CAD build for the part. Positions are in the model's coordinates, mm. A direction names the side the tool comes from. Give positions to 0.01 mm unless a question says otherwise; leave off trailing zeros. Write each loop counter-clockwise with the first axis right and the second up, starting at its lowest first coordinate (ties: lowest second). Pieces come first, ordered by that corner, then holes. Notation, with made-up numbers: (25, -16.75) -> (31, -16.75) arc R21 cw to (31, 13.25) -> close; hole circle Ø4 at (15, 21.5). An arc over 180 degrees is marked (long way). Answer as a JSON object with one key per item and string values.
Autodesk Inventor part; units mm, degrees
ref_plane "YZ Plane" through (0, 0, 0) normal (1, 0, 0) x (0, 1, 0)
ref_plane "XZ Plane" through (0, 0, 0) normal (0, 1, 0) x (-1, 0, 0)
ref_plane "XY Plane" through (0, 0, 0) normal (0, 0, 1) x (1, 0, 0)
sketch "Sketch1" plane through (0, 0, 0) normal (0, 1, 0) x (-1, 0, 0)
  circle A0 centre (0, 0.2739) radius 5
  point P0 (0, 0)
  dimension "d0" = 10
extrude "Extrusion1" add sketch "Sketch1" along normal blind 28
sketch "Sketch3" plane through (0, 28, 0.2739) normal (0, 1, 0) x (1, 0, 0)
  line L0 (14, -5.25) -> (-14, -5.25)
  line L1 (-14, -5.25) -> (-14, 5.25)
  line L2 (-14, 5.25) -> (14, 5.25)
  line L3 (14, 5.25) -> (14, -5.25)
  line L4 (14, -5.25) -> (-14, 5.25) construction
  line L5 (-14, -5.25) -> (14, 5.25) construction
  circle A0 centre (0, 0) radius 5
  point P0 (0, 0.2739)
  point P1 (0, 0)
  dimension "d5" = 28
  dimension "d6" = 10.5
  dimension "d16" = 5.25
extrude "Extrusion2" add sketch "Sketch3" along normal blind 34 contours L0 L1 L2 L3 | A0
sketch "Sketch4" plane through (-14, 28, 5.5239) normal (0, 0, 1) x (1, 0, 0)
  circle A0 centre (14, 20) radius 7.5
  line L0 (9, -28) -> (19, -28)
  line L1 (28, 0) -> (28, 34)
  circle A1 centre (14, 20) radius 14
  line L2 (19, 0) -> (9, 0)
  line L3 (9, 0) -> (1.7243, 13.2689)
  line L4 (19, -28) -> (19, 0)
  line L5 (19, 0) -> (26.2757, 13.2689)
  line L6 (19, 0) -> (28, 0)
  line L7 (28, 0) -> (28, 20)
  line L8 (28, 0) -> (0, 0)
  line L9 (0, 0) -> (9, 0)
  line L10 (0, 0) -> (0, 20)
  line L11 (0, 0) -> (0, 34)
  line L12 (0, 20) -> (0, 34)
  line L13 (0, 34) -> (14, 34)
  line L14 (0, 34) -> (28, 34)
  line L15 (14, 34) -> (28, 34)
  line L16 (28, 34) -> (28, 20)
  point P0 (14, -28)
  dimension "d9" = 15
  dimension "d10" = 48
  dimension "d11" = 14
  dimension "d12" = 28
  dimension "d13" = 13.2689
extrude "Extrusion3" cut sketch "Sketch4" against normal blind 34 contours A0 | L6 L5 A1 L1 | A1 L14 L1 | A1 L11 L13 | L8 L10 A1 L3
properties part number "K"
1) 3-axis set-ups, long thin cutter, end or side, ignore diameter. For faces 1 (the cylindrical face through (1.084, 13.804, 5.155)), 2 (the flat face through (3.3, 41, 5.524)): which of +Z, -Z, +X, -X, +Y, -Y reach the whole face in a straight line?
Model answer:
{"face 1": "-Y", "face 2": "+Z, +X, -X, +Y, -Y"}
2) Slice it at A-A (x = 0). List the corners of the cut face in (y, z), then the cut area to 4 significant figures.
Model answer:
{"outline": "(0, -4.73) -> (28, -4.73) -> (28, -4.98) -> (40.5, -4.98) -> (40.5, 5.52) -> (28, 5.52) -> (28, 5.27) -> (0, 5.27) -> close; (55.5, -4.98) -> (62, -4.98) -> (62, 5.52) -> (55.5, 5.52) -> close", "area": "479.5 mm2"}
3) Wall check: probe 1 along Y at (x, z) = (0, 0); probe 2 along Y at (x, z) = (5.5, -1.75); probe 3 along X at (y, z) = (51, 4.5). Give the ranges that are in metal, low to high.
Model answer:
{"probe 1": "y = 0 to 40.5, 55.5 to 62", "probe 2": "y = 28.91 to 42.9, 53.1 to 60.87", "probe 3": "x = -13.67 to -6.87, 6.87 to 13.67"}
4) Slice it at C-C (z = 3.5). List the corners of the cut face in (x, y).
Model answer:
{"outline": "(-12.28, 41.27) -> (-5, 28) -> (-3.82, 28) -> (-3.82, 0) -> (3.82, 0) -> (3.82, 28) -> (5, 28) -> (12.28, 41.27) arc R14 ccw (long way) to start; hole circle Ø15 at (0, 48)"}
5) Mould opens along X. For faces 3 (the flat face through (8.587, 34.542, 0.347)), 4 (the cylindrical face through (0, 62, 0)), 5 (the cylindrical face through (-1.63, 40.68, 0.35)), 6 (the flat face through (-1.5, 28, 5.22)) say: released by +X, released by -X, zero draft, split by the parting line, or undercut.
Model answer:
{"face 3": "released by +X", "face 4": "split by the parting line", "face 5": "undercut", "face 6": "zero draft"}
6) Pin check, flat tips, straight feed: pin 1 (1.5 mm diameter, centred on x = -7, z = 4, fed in from +Y); pin 2 (1 mm diameter, centred on y = 26, z = -1, fed in from -X); pin 3 (10 mm diameter, centred on x = -2.5, y = 11.5, fed in from +Z). Stop position of each tip, or through.
Model answer:
{"pin 1": "stops at y = 60.53", "pin 2": "stops at x = -4.94", "pin 3": "stops at z = 5.27"}
7) Slice it at B-B (y = 48). List the corners of the cut face in (x, z).
Model answer:
{"outline": "(-14, -4.98) -> (-7.5, -4.98) -> (-7.5, 5.52) -> (-14, 5.52) -> close; (7.5, -4.98) -> (14, -4.98) -> (14, 5.52) -> (7.5, 5.52) -> close"}
8) Slice it at D-D (x = -3). List the corners of the cut face in (y, z), then the cut area to 3 significant figures.
Model answer:
{"outline": "(0, -3.73) -> (28, -3.73) -> (28, -4.98) -> (41.13, -4.98) -> (41.13, 5.52) -> (28, 5.52) -> (28, 4.27) -> (0, 4.27) -> close; (54.87, -4.98) -> (61.67, -4.98) -> (61.67, 5.52) -> (54.87, 5.52) -> close", "area": "433 mm2"}
